Could you check a few things on this model? Use its own coordinates, in mm. Round coordinates to 2 decimals unless told otherwise and drop trailing zeros. Write each loop counter-clockwise with the first axis right and the second up, starting at its lowest first coordinate (ties: lowest second). Pieces come first, ordered by that corner, then holes. Notation, with made-up numbers: (12.25, 89.5) - (31.25, 89.5) arc R34 cw to (31.25, 121.5) - close; hole circle Ø9 at (65, 19). An arc over 180 degrees is marked (long way). Put each result on its own line as item: value.
from build123d import *

# Parameters (mm, degrees)
SKETCH_1_W          = 47
SKETCH_1_H          = 28
EXTRUDE_1_DEPTH     = 12
SKETCH_2_R          = 2
CUT_EXTRUDE_1_DEPTH = 12


with BuildPart() as part:
    # 草图1 → 凸台-拉伸1 (new body)
    with BuildSketch(Plane.XY):
        with Locations((-10.441605839, 22.569343066)):
            Rectangle(SKETCH_1_W, SKETCH_1_H)
    extrude(amount=EXTRUDE_1_DEPTH)

    # 草图2 → 切除-拉伸1 (cut)
    with BuildSketch(Plane.XY.offset(12)):
        with Locations((-19.691605839, 31.819343066)):
            Circle(SKETCH_2_R)
        with Locations(Location((-1.191605839, 31.819343066, 0), (0, 0, 180))):
            Circle(SKETCH_2_R)
        with Locations((-1.191605839, 13.319343066)):
            Circle(SKETCH_2_R)
        with Locations(Location((-19.691605839, 13.319343066, 0), (0, 0, 180))):
            Circle(SKETCH_2_R)
    extrude(amount=-CUT_EXTRUDE_1_DEPTH, mode=Mode.SUBTRACT)


solid = part.part
(1) Please list where these lines run through material, in increasing order: probe 1 along X at (y, z) = (14.25, 0.5); probe 2 along Y at (x, z) = (-21, 1.75); probe 3 along X at (y, z) = (11.75, 2.75). Write a range as from..to.
Values found:
probe 1: x = -33.94..-21.46, -17.92..-2.96, 0.58..13.06
probe 2: y = 8.57..11.81, 14.83..30.31, 33.33..36.57
probe 3: x = -33.94..-20.93, -18.45..-2.43, 0.05..13.06
(2) If we mould it in two halves opening along Y, with no side actions, what happens to faces 1 (the face through (-11, 36.569, 6)), 2 (the face through (-11, 23, 0)), 3 (the face through (-18.104, 14.536, 6.084)), 4 (the face through (-2.267, 30.133, 6.084))? For each: pulls with the +Y half, pulls with the -Y half, needs draft (parallel to the pull), parting line crosses it, or undercut.
Values found:
face 1: pulls with the +Y half
face 2: needs draft
face 3: undercut
face 4: undercut
(3) Imagine slicing it at A-A, the plane y = 32.5. List the corners of the cut face in (x, z) for me.
Values found:
outline: (-33.94, 0) - (-21.57, 0) - (-21.57, 12) - (-33.94, 12) - close; (-17.81, 0) - (-3.07, 0) - (-3.07, 12) - (-17.81, 12) - close; (0.69, 0) - (13.06, 0) - (13.06, 12) - (0.69, 12) - close
(4) Imagine slicing it at B-B, the plane z = 2.75. List the corners of the cut face in (x, y) for me.
Values found:
outline: (-33.94, 8.57) - (13.06, 8.57) - (13.06, 36.57) - (-33.94, 36.57) - close; hole circle Ø4 at (-19.69, 13.32); hole circle Ø4 at (-19.69, 31.82); hole circle Ø4 at (-1.19, 13.32); hole circle Ø4 at (-1.19, 31.82)
